```python
from build123d import *

# Parameters (mm, degrees)
EXTRUDE_1_DEPTH     = 10
SKETCH_4_W          = 25
SKETCH_4_H          = 14
CUT_EXTRUDE_1_DEPTH = 25
LOFT_START          = 2
LOFT_2_DEPTH        = 4
EXTRUDE_2_DEPTH     = 2
CUT_EXTRUDE_2_DEPTH = 33.86335345
LOFT_START_2        = -2
LOFT_4_DEPTH        = 4


# Read off the part's stored shape, not the designer's step: 切除-放样2, 放样4
with BuildPart() as part:
    # Sketch 1 → 凸台-拉伸1 (new, symmetric)
    with BuildSketch(Plane.XY):
        Polygon((-14, -8), (-8, -8), (8, 8), (8, 14), (14, 14), (14, -14), (-14, -14), align=None)
    extrude(amount=EXTRUDE_1_DEPTH, both=True)

    # 草图4 → 切除-拉伸1 (cut)
    with BuildSketch(Plane(origin=(0, 14, 0), x_dir=(1, 0, 0), z_dir=(0, 1, 0))):
        with Locations((-1.5, 0)):
            Rectangle(SKETCH_4_W, SKETCH_4_H)
    extrude(amount=-CUT_EXTRUDE_1_DEPTH, mode=Mode.SUBTRACT)

    # Sketch 1 2 → 切除-放样1 section 0
    with BuildSketch(Plane(origin=(12.5, 0, 0), x_dir=(0, 0, -1), z_dir=(1, 0, 0))):
        with BuildLine():
            Line((6, 10), (6, 12.5))
            Line((6, 12.5), (2, 12.5))
            Line((2, 12.5), (2, 10))
            Line((2, 10), (6, 10))
        make_face()
    # 草图2<110> → 切除-放样1 section 1
    with BuildSketch(Plane(origin=(14, 0, 0), x_dir=(0, 0, -1), z_dir=(1, 0, 0))):
        with BuildLine():
            Line((2, 8.5), (6, 8.5))
            Line((6, 8.5), (6, 12.5))
            Line((6, 12.5), (2, 12.5))
            Line((2, 12.5), (2, 8.5))
        make_face()
    loft_1 = loft(mode=Mode.SUBTRACT)

    # 切除-放样2 outline → 切除-放样2 (cut)
    with BuildSketch(Plane.XY.offset(LOFT_START)):
        Polygon((12.5, 12.5), (12.5, 10), (14, 8.5), (14, 12.5), align=None)
    loft_2 = extrude(amount=LOFT_2_DEPTH, mode=Mode.SUBTRACT)

    # 基准面1草图<9> → 切除-放样3 section 0
    with BuildSketch(Plane(origin=(12.5, 0, 0), x_dir=(0, 0, -1), z_dir=(1, 0, 0))):
        with BuildLine():
            Line((-6, -4), (6, -4))
            Line((6, -4), (6, -7.5))
            Line((6, -7.5), (-6, -7.5))
            Line((-6, -7.5), (-6, -4))
        make_face()
    # 草图2<114> → 切除-放样3 section 1
    with BuildSketch(Plane(origin=(14, 0, 0), x_dir=(0, 0, -1), z_dir=(1, 0, 0))):
        with BuildLine():
            Line((-6, -4), (6, -4))
            Line((6, -4), (6, -9))
            Line((6, -9), (-6, -9))
            Line((-6, -9), (-6, -4))
        make_face()
    loft_3 = loft(mode=Mode.SUBTRACT)

    # 草图9 → 凸台-拉伸2 (add, symmetric)
    with BuildSketch(Plane.XY):
        Polygon((15, -8), (15, -9), (12.5, -9), (12.5, -6.5), align=None)
    extrude_2 = extrude(amount=EXTRUDE_2_DEPTH, both=True)

    # 草图2<115> → 切除-拉伸2 (cut, through all)
    with BuildSketch(Plane(origin=(14, 0, 0), x_dir=(0, 0, -1), z_dir=(1, 0, 0))):
        with BuildLine():
            Line((-3.25, 0.25), (-3.25, 5.75))
            ThreePointArc((-3.25, 5.75), (0, 9), (3.25, 5.75))
            Line((3.25, 5.75), (3.25, 0.25))
            ThreePointArc((3.25, 0.25), (0, -3), (-3.25, 0.25))
        make_face()
    cut_extrude_2 = extrude(amount=-CUT_EXTRUDE_2_DEPTH, mode=Mode.SUBTRACT)

    # 放样4 outline → 放样4 (add)
    with BuildSketch(Plane.XY.offset(LOFT_START_2)):
        Polygon((14, 10.5), (15, 10.5), (15, 11.5), (14, 12.5), align=None)
    loft_4 = extrude(amount=LOFT_4_DEPTH)

    # 镜向1: 切除-放样1, 切除-放样2, 切除-放样3, 凸台-拉伸2, 切除-拉伸2, 放样4 across plane
    add(loft_1.mirror(Plane(origin=(0, 0, 0), x_dir=(0, 0, 1), z_dir=(0.7071067811865474, 0.7071067811865477, 0))), mode=Mode.SUBTRACT)
    add(loft_2.mirror(Plane(origin=(0, 0, 0), x_dir=(0, 0, 1), z_dir=(0.7071067811865474, 0.7071067811865477, 0))), mode=Mode.SUBTRACT)
    add(loft_3.mirror(Plane(origin=(0, 0, 0), x_dir=(0, 0, 1), z_dir=(0.7071067811865474, 0.7071067811865477, 0))), mode=Mode.SUBTRACT)
    add(extrude_2.mirror(Plane(origin=(0, 0, 0), x_dir=(0, 0, 1), z_dir=(0.7071067811865474, 0.7071067811865477, 0))))
    add(cut_extrude_2.mirror(Plane(origin=(0, 0, 0), x_dir=(0, 0, 1), z_dir=(0.7071067811865474, 0.7071067811865477, 0))), mode=Mode.SUBTRACT)
    add(loft_4.mirror(Plane(origin=(0, 0, 0), x_dir=(0, 0, 1), z_dir=(0.7071067811865474, 0.7071067811865477, 0))))


solid = part.part
```
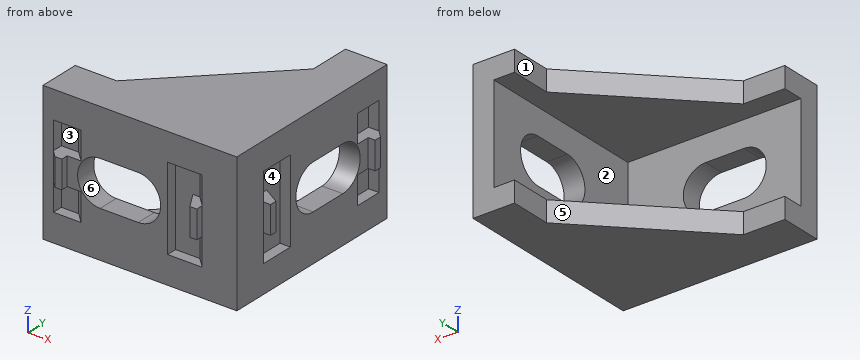
Build history of the part. All positions in model axes, mm. Face numbers are marked on the shaded views. A direction names the side the tool comes from. Give positions to 0.01 mm unless a question says otherwise; leave off trailing zeros. Loops run counter-clockwise (first coordinate to the right, second up) from the corner with the lowest first, then second, coordinate; pieces in that order, holes last. Notation, with made-up numbers: (65, 78) -> (107, 78) arc R15 ccw to (107, 84) -> close; hole circle Ø3 at (50.5, 34). An arc over 180 degrees is marked (long way). One line per question, with ' | ' between items.
Q1. Pull direction Y, two halves, no side cores. Call the marked faces 4, 5 and 6: pulls with the +Y half, pulls with the -Y half, needs draft (parallel to the pull), parting line crosses it, or undercut.
Filled sheet:
face 4: undercut | face 5: pulls with the +Y half | face 6: needs draft
Q2. Tool access for the marked faces 1, 2 and 3: list every direction of +Z, -Z, +X, -X, +Y, -Y with a clear straight run to the whole face (end or side of a thin tool).
Filled sheet:
face 1: +Z, -Z, -X, +Y | face 2: -X, +Y | face 3: -Y
Q3. Cut at A-A, the plane x = -1. Write the cut outline in (y, z), plus the area to 4 significant figures.
Filled sheet:
outline: (-14, -10) -> (-1, -10) -> (-1, -7) -> (-11, -7) -> (-11, -3.25) -> (-14, -3.25) -> close; (-14, 3.25) -> (-11, 3.25) -> (-11, 7) -> (-1, 7) -> (-1, 10) -> (-14, 10) -> close | area: 100.5 mm²
Q4. Drop flat-ended pins along their axis: pin 1 (4 mm diameter, centred on y = 2.5, z = 7.5, fed in from -X); pin 2 (1 mm diameter, centred on x = 5, z = 2.5, fed in from -Y); pin 3 (7.5 mm diameter, centred on x = -7.5, y = 0, fed in from +Z); pin 4 (6 mm diameter, centred on y = 5.5, z = 1, fed in from -X). Give the stop position or say it passes through.
Filled sheet:
pin 1: stops at x = 0.5 | pin 2: stops at y = -12.5 | pin 3: passes through | pin 4: stops at x = 11
Q5. Cut at D-D, the plane x = 10. Write the cut outline in (y, z).
Filled sheet:
outline: (-14, -10) -> (14, -10) -> (14, -7) -> (-11, -7) -> (-11, 7) -> (14, 7) -> (14, 10) -> (-14, 10) -> close
Q6. Cut at C-C, the plane z = 5.5. Write the cut outline in (x, y).
Filled sheet:
outline: (-14, -14) -> (-12.5, -14) -> (-12.5, -12.5) -> (-10, -12.5) -> (-8.5, -14) -> (4, -14) -> (4, -12.5) -> (7.5, -12.5) -> (9, -14) -> (14, -14) -> (14, -9) -> (12.5, -7.5) -> (12.5, -4) -> (14, -4) -> (14, 8.5) -> (12.5, 10) -> (12.5, 12.5) -> (14, 12.5) -> (14, 14) -> (11, 14) -> (11, -11) -> (-14, -11) -> close
Q7. Drill centre lines: line 1 along Z through (x, y) = (13.25, 5); line 2 along Z through (x, y) = (9.25, -2.75); line 3 along Y through (x, z) = (-4, 5.5). Where is each one in solid material? Low to high. Write a range as [from, to].
Filled sheet:
line 1: z = [-10, -3.25], [3.25, 10] | line 2: z = [-10, -7], [7, 10] | line 3: y = [-14, -11]
Q8. Cut at B-B, the plane z = 0. Count the separate pieces of the cut face and the enclosed holes in it, plus the area to 4 significant figures.
Filled sheet:
separate pieces: 3 | enclosed holes: 0 | area: 83.75 mm²
